```python
from build123d import *

# Parameters (mm, degrees)
SKETCH1_W           = 51
SKETCH1_H           = 78
BOSS_EXTRUDE1_DEPTH = 3
SKETCH2_W           = 10
SKETCH2_H           = 30
BOSS_EXTRUDE3_DEPTH = 6
SKETCH3_W           = 6
SKETCH3_H           = 24
CUT_EXTRUDE1_DEPTH  = 31.5
BOSS_EXTRUDE4_REACH = 53


with BuildPart() as part:
    # Sketch1 → Boss-Extrude1 (new body)
    with BuildSketch(Plane.XY):
        with Locations((-25.5, 39)):
            Rectangle(SKETCH1_W, SKETCH1_H)
    extrude(amount=BOSS_EXTRUDE1_DEPTH)

    # Sketch2 → Boss-Extrude3 (add)
    with BuildSketch(Plane.XY.offset(3)):
        with Locations((-25.5, 39)):
            Rectangle(SKETCH2_W, SKETCH2_H)
    extrude(amount=BOSS_EXTRUDE3_DEPTH)

    # Sketch3 → Cut-Extrude1 (cut, through all)
    with BuildSketch(Plane.ZY.offset(30.5)):
        with Locations((6, 39)):
            Rectangle(SKETCH3_W, SKETCH3_H)
    extrude(amount=-CUT_EXTRUDE1_DEPTH, mode=Mode.SUBTRACT)

    # Sketch5 → Boss-Extrude4 (add, up to next)
    with BuildSketch(Plane.XZ.offset(-51), mode=Mode.PRIVATE) as boss_extrude4_sk1:
        Polygon((-30.5, 9), (-20.5, 9), (-20.5, 8), (-25, 4), (-25, 3), (-26, 3), (-26, 4), (-30.5, 8), align=None)
    boss_extrude4_tool1 = extrude(boss_extrude4_sk1.sketch, amount=BOSS_EXTRUDE4_REACH, mode=Mode.PRIVATE) - part.part
    add(boss_extrude4_tool1.solids().sort_by_distance((-25.5, 51, 7.045455))[0])


solid = part.part
```
For this review, take the finished solid that the model builds, in its own axes (mm). A direction names the side the tool comes from. Give positions to 0.01 mm unless a question says otherwise; leave off trailing zeros. Order: outer loops, then holes, each group sorted by start corner. A loop starts at its lowest first (then second) coordinate and runs counter-clockwise, first axis right, second up.
1) Insertion check: pin 1 (5 mm diameter, centred on x = -25, z = 6, fed in from -Y); pin 2 (3.5 mm diameter, centred on x = -23, z = 6.5, fed in from +Y); pin 3 (0.5 mm diameter, centred on y = 38.5, z = 3.5, fed in from +X). Each pin has a flat end and moves straight along its axis. Give the tip position at first contact, or say it passes through.
2) Take a section at A-A (z = 6). Give the boundary of the cut face in (x, y).
3) Take a section at D-D (y = 61.5). Give the boundary of the cut face in (x, z).
4) Wall thickness on line 1 (Y direction, x = -30, z = 5.5); line 2 (Z direction, x = -49, y = 39.5); line 3 (X direction, y = 53.5, z = 5.5): over which ranges is each line inside the solid? List them lowest first.
5) Take a section at C-C (x = -6). Give the boundary of the cut face in (y, z), then the cut area to 3 significant figures.
6) The part is to be moulded in two halves that separate along Z. For faces 1 (the face through (-29, 27, 5)), 2 (the face through (-20.5, 39.2, 8.7)), 3 (the face through (-22, 27, 5)), 4 (the face through (-26, 39, 9)), say which applies: released by +Z, released by -Z, zero draft, split by the parting line, or undercut.
7) Take a section at B-B (y = 46). Give the boundary of the cut face in (x, z), then the cut area to 3 significant figures.
8) For faces 5 (the face through (-28.218, 39.168, 5.972)), 6 (the face through (-22.718, 39.168, 6.028)), 7 (the face through (-26, 54, 6)), list the 3-axis set-ups (+Z, -Z, +X, -X, +Y, -Y) from which the entire face can be reached by the end or side of a thin tool; tool diameter is ignored.
Derived:
1. pin 1: stops at y = 24
1. pin 2: stops at y = 54
1. pin 3: stops at x = -25
2. outline: (-30.5, 24) - (-20.5, 24) - (-20.5, 27) - (-22.75, 27) - (-22.75, 51) - (-20.5, 51) - (-20.5, 54) - (-30.5, 54) - (-30.5, 51) - (-28.25, 51) - (-28.25, 27) - (-30.5, 27) - close
3. outline: (-51, 0) - (0, 0) - (0, 3) - (-51, 3) - close
4. line 1: y = 24 to 27, 51 to 54
4. line 2: z = 0 to 3
4. line 3: x = -30.5 to -20.5
5. outline: (0, 0) - (78, 0) - (78, 3) - (0, 3) - close
5. area: 234 mm2
6. face 1: undercut
6. face 2: zero draft
6. face 3: undercut
6. face 4: released by +Z
7. outline: (-51, 0) - (0, 0) - (0, 3) - (-25, 3) - (-25, 4) - (-20.5, 8) - (-20.5, 9) - (-30.5, 9) - (-30.5, 8) - (-26, 4) - (-26, 3) - (-51, 3) - close
7. area: 186 mm2
8. face 5: -X
8. face 6: +X
8. face 7: +Z, +X, -X, +Y
